Verification items for the finished model (mm, model axes). Face numbers are marked on the shaded views. A direction names the side the tool comes from. Round coordinates to 2 decimals unless told otherwise and drop trailing zeros. Order: outer loops, then holes, each group sorted by start corner. A loop starts at its lowest first (then second) coordinate and runs counter-clockwise, first axis right, second up. Notation, with made-up numbers: M 66,36.25 L 106,36.25 A12 cw 106,56.25 Z; hole C -34,46.5 d9. An arc over 180 degrees is marked long. Use CSV: the item, a comma, the result in double quotes. Start each with the question number.
Q1. Sectioned sample at A-A (y = 39). Enter the section's corners in (x, z), and give its area (3 significant figures).
Q2. Sectioned sample at D-D (z = 132). Enter the section's corners in (x, y), and give its area (3 significant figures).
Q3. Gauge pin test, flat ends, axial feed: pin 1 Ø12 at (y, z) = (67.5, 127.5) entering from +X; pin 2 Ø1.5 at (y, z) = (23.5, 21) entering from -X; pin 3 Ø1 at (x, y) = (137, 43.5) entering from +Z. Record the tip position at first contact, or that the pin passes through.
Q4. Sectioned sample at B-B (x = 29). Enter the section's corners in (y, z), and give its area (3 significant figures).
Q5. Scan lines: line 1 (Z direction, x = 12, y = 44); line 2 (Z direction, x = 118.5, y = 47.5); line 3 (Y direction, x = 33.5, z = 97). Record each from-to range of solid material in increasing order.
Q6. Set-up check for the marked faces 1, 2, 3 and 4: record each of +Z, -Z, +X, -X, +Y, -Y from which the full face is reachable in a straight line by a thin tool's end or side.
Q7. Sectioned sample at C-C (y = 58.5). Enter the section's corners in (x, z).
Q8. Mould release check, pull along Z, two halves, no side actions. Record for the marked faces 5, 6, 7 and 8: +Z half, -Z half, draft (parallel to the pull), parting line (faces both ways), or undercut.
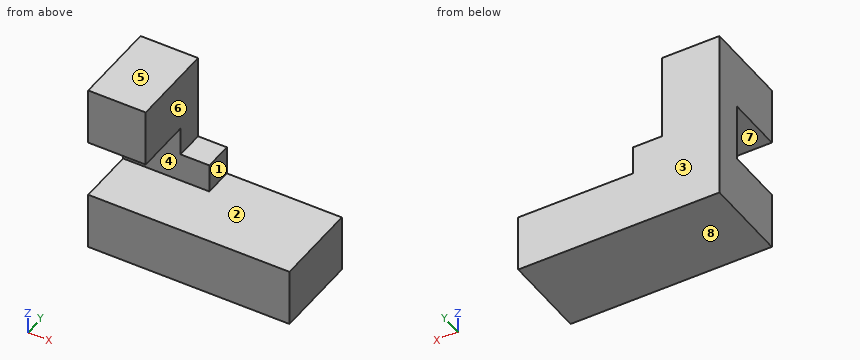
```python
from build123d import *

# Parameters (mm, degrees)
F0_W     = 177.8
F0_H     = 76.2
F1_DEPTH = 50.8
F2_W     = 76.2
F2_H     = 25.4
F3_DEPTH = 25.4
F4_W     = 50.8
F4_H     = 25.4
F5_DEPTH = 76.2
F6_W     = 50.8
F6_H     = 50.8
F7_DEPTH = 50.8


with BuildPart() as f1:
    # F0 (on Top) → F1 (new body)
    with BuildSketch(Plane.XY):
        with Locations((88.9, 38.1)):
            Rectangle(F0_W, F0_H)
    extrude(amount=F1_DEPTH)

    # F2 (on face) → F3 (join)
    with BuildSketch(Plane.XY.offset(50.8)):
        with Locations((38.1, 63.5)):
            Rectangle(F2_W, F2_H)
    extrude(amount=F3_DEPTH)

    # F4 (on face) → F5 (join)
    with BuildSketch(Plane.XY.offset(76.2)):
        with Locations((25.4, 63.5)):
            Rectangle(F4_W, F4_H)
    extrude(amount=F5_DEPTH)

    # F6 (on face) → F7 (join)
    with BuildSketch(Plane.XZ.offset(-50.8)):
        with Locations((25.4, 127)):
            Rectangle(F6_W, F6_H)
    extrude(amount=F7_DEPTH)


solid = f1.part
```
Verdict:
1,outline,"M 0,0 L 177.8,0 L 177.8,50.8 L 0,50.8 Z; M 0,101.6 L 50.8,101.6 L 50.8,152.4 L 0,152.4 Z"
1,area,"11,600 mm²"
2,outline,"M 0,0 L 50.8,0 L 50.8,76.2 L 0,76.2 Z"
2,area,"3,870 mm²"
3,pin 1,"stops at x = 50.8"
3,pin 2,"stops at x = 0"
3,pin 3,"stops at z = 50.8"
4,outline,"M 0,0 L 76.2,0 L 76.2,152.4 L 0,152.4 L 0,101.6 L 50.8,101.6 L 50.8,50.8 L 0,50.8 Z"
4,area,"9,030 mm²"
5,line 1,"z = 0 to 50.8, 101.6 to 152.4"
5,line 2,"z = 0 to 50.8"
5,line 3,"y = 50.8 to 76.2"
6,face 1,"+Z, +X, +Y, -Y"
6,face 2,"+X, -Y"
6,face 3,"+Z, -Z, +X, -X, +Y"
6,face 4,"+X, -X, -Y"
7,outline,"M 0,0 L 177.8,0 L 177.8,50.8 L 76.2,50.8 L 76.2,76.2 L 50.8,76.2 L 50.8,152.4 L 0,152.4 Z"
8,face 5,"+Z half"
8,face 6,"draft"
8,face 7,"undercut"
8,face 8,"-Z half"
